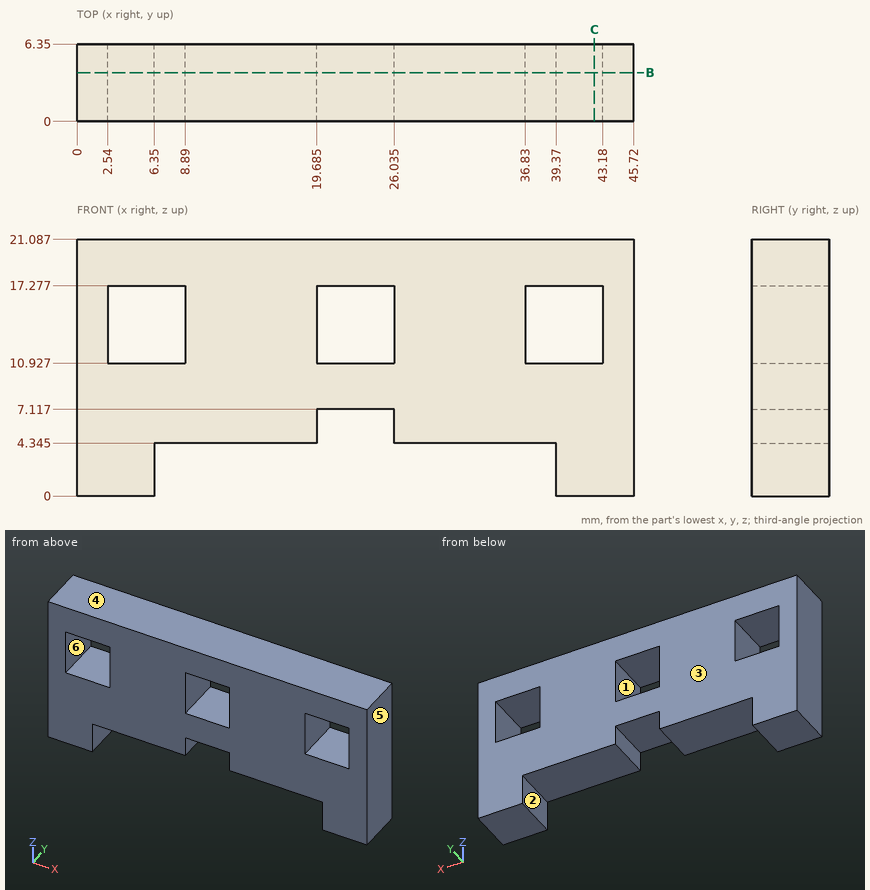
Source: three-view drawing plus pictorial views. Frame: mm from the lowest corner of the part. A direction names the side the tool comes from. Round coordinates to 2 decimals unless told otherwise and drop trailing zeros. Order: outer loops, then holes, each group sorted by start corner. A loop starts at its lowest first (then second) coordinate and runs counter-clockwise, first axis right, second up. Notation, with made-up numbers: M 32.25,-8.75 L 66.25,-8.75 A32 cw 66.25,21.25 Z; hole C -19,76 d8. An arc over 180 degrees is marked long. One line per item, written item: value.
(1) Line query: probe 1 along X at (y, z) = (1.75, 13.5) (1 decimal); probe 2 along X at (y, z) = (5, 6.75) (1 decimal); probe 3 along Z at (x, y) = (23.5, 2.5). Output: solid intervals per line, ascending. Write a range as [from, to].
Result sheet:
probe 1: [0, 2.5], [8.9, 19.7], [26, 36.8], [43.2, 45.7]
probe 2: [0, 19.7], [26, 45.7]
probe 3: [7.12, 10.93], [17.28, 21.09]
(2) Pull-direction query (Z, two-part tool) for the marked faces 4, 5 and 6; classes: pulls with the +Z half, pulls with the -Z half, needs draft (parallel to the pull), parting line crosses it, or undercut.
Result sheet:
face 4: pulls with the +Z half
face 5: needs draft
face 6: undercut
(3) Cut plane C-C (x = 42.5). Return the cut outline in (y, z).
Result sheet:
outline: M 0,0 L 6.35,0 L 6.35,10.93 L 0,10.93 Z; M 0,17.28 L 6.35,17.28 L 6.35,21.09 L 0,21.09 Z
(4) Cut plane B-B (y = 4). Give the number of separate pieces and of enclosed holes in the cut face, and give its area (3 significant figures).
Result sheet:
separate pieces: 1
enclosed holes: 3
area: 682 mm2
(5) Reachability of the marked faces 1, 2 and 3 from +Z, -Z, +X, -X, +Y, -Y: full face, straight path, thin tool, end or side. Return the list, or none.
Result sheet:
face 1: +Y, -Y
face 2: -Z, +Y, -Y
face 3: +Z, -Z, +X, -X, +Y
(6) Pin query (flat end, axial travel): P1, Ø1.9, axis at x = 21.5, y = 3.5, coming from the -Z side. Return the tip coordinate at first contact, or that it passes through.
Result sheet:
P1: z = 7.12
